```python
from build123d import *

# Parameters (mm, degrees)
F0_R      = 25.4
F1_DEPTH  = 95.25
F2_R      = 25.4
F2_R_2    = 19.05
F3_DEPTH  = 38.1
F4_R      = 25.4
F4_R_2    = 19.05
F5_DEPTH  = 38.1
F7_DEPTH  = 12.7
F9_DEPTH  = 46.228
F10_R     = 4.826
F11_DEPTH = 22.352


with BuildPart() as f1:
    # F0 (on Right) → F1 (new body)
    with BuildSketch(Plane.YZ):
        Circle(F0_R)
    extrude(amount=F1_DEPTH)

    # F2 (on face) → F3 (cut)
    with BuildSketch(Plane.YZ.offset(95.25)):
        Circle(F2_R)
        Circle(F2_R_2, mode=Mode.SUBTRACT)
    extrude(amount=-F3_DEPTH, mode=Mode.SUBTRACT)

    # F4 (on face) → F5 (cut)
    with BuildSketch(Plane(origin=(0, 0, 0), x_dir=(0, -1, 0), z_dir=(-1, 0, 0))):
        Circle(F4_R)
        Circle(F4_R_2, mode=Mode.SUBTRACT)
    extrude(amount=-F5_DEPTH, mode=Mode.SUBTRACT)

    # F6 (on face) → F7 (cut)
    with BuildSketch(Plane(origin=(0, 0, 0), x_dir=(0, -1, 0), z_dir=(-1, 0, 0))):
        with BuildLine():
            ThreePointArc((6.35, 17.9605122421), (3.2213926947, 18.7756525614), (0, 19.05))
            ThreePointArc((0, 19.05), (-3.2213926947, 18.7756525614), (-6.35, 17.9605122421))
            Line((-6.35, 17.9605122421), (-6.35, -17.9605122421))
            ThreePointArc((-6.35, -17.9605122421), (-3.2213926947, -18.7756525614), (0, -19.05))
            ThreePointArc((0, -19.05), (3.2213926947, -18.7756525614), (6.35, -17.9605122421))
            Line((6.35, -17.9605122421), (6.35, 17.9605122421))
        make_face()
    extrude(amount=-F7_DEPTH, mode=Mode.SUBTRACT)

    # F8 (on face) → F9 (cut)
    with BuildSketch(Plane.YZ.offset(95.25)):
        with BuildLine():
            Line((-40.058898566, 25.4), (-40.058898566, 21.5428465581))
            Line((-40.058898566, 21.5428465581), (-40.058898566, 12.7))
            Line((-40.058898566, 12.7), (-14.1990316571, 12.7))
            ThreePointArc((-14.1990316571, 12.7), (0, 19.05), (14.1990316571, 12.7))
            Line((14.1990316571, 12.7), (36.141101434, 12.7))
            Line((36.141101434, 12.7), (36.141101434, 25.4))
            Line((36.141101434, 25.4), (-40.058898566, 25.4))
        make_face()
        with BuildLine():
            ThreePointArc((14.1990316571, 12.7), (0, 19.05), (-14.1990316571, 12.7))
            Line((-14.1990316571, 12.7), (14.1990316571, 12.7))
        make_face()
    extrude(amount=-F9_DEPTH, mode=Mode.SUBTRACT)

    # F10 (on face) → F11 (cut)
    with BuildSketch(Plane.XY.offset(12.7)):
        with Locations((76.2, 0)):
            Circle(F10_R)
    extrude(amount=-F11_DEPTH, mode=Mode.SUBTRACT)


solid = f1.part
```
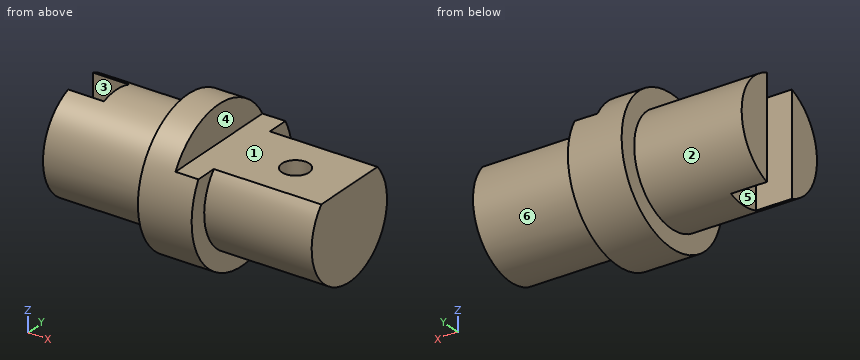
Read the model definition and answer for the solid it produces. Units are mm, in the model's axes. Face numbers are marked on the shaded views. A direction names the side the tool comes from. Give positions to 0.01 mm unless a question says otherwise; leave off trailing zeros. Loops run counter-clockwise (first coordinate to the right, second up) from the corner with the lowest first, then second, coordinate; pieces in that order, holes last.
Item 1: The part is cut by section A-A (z = 0). Write down the section's boundary in (x, y).
Item 2: For the marked faces 4, 5 and 6, determine the directions among +Z, -Z, +X, -X, +Y, -Y from which every point of the face is accessible in a straight line to the end or side of a thin tool.
Item 3: Each of these flat-tipped pins is pushed along its axis until it touches: pin 1 Ø8.5 at (x, y) = (76.2, 0) entering from +Z; pin 2 Ø14 at (x, z) = (3.5, 0) entering from -Y; pin 3 Ø10.5 at (x, y) = (77, -1) entering from +Z. Where does it stop, or does it pass through?
Item 4: Find the intervals of material crossed by line 1 along X through (y, z) = (21.5, -3); line 2 along Y through (x, z) = (15, -0.5); line 3 along Y through (x, z) = (76, -4), in increasing order.
Item 5: The part is cut by section C-C (y = 0). Write down the section's boundary in (x, z).
Item 6: The mould has two halves that part along Y. Classify the marked faces 1, 2 and 3: released by +Y, released by -Y, zero draft, split by the parting line, or undercut.
Item 7: The part is cut by section D-D (z = -11.5). Write down the section's boundary in (x, y), and give its area (3 significant figures).
Item 8: The part is cut by section B-B (x = 7.5). Write down the section's boundary in (y, z), and give its area (3 significant figures).
Taken from the geometry:
1. outline: (0, -19.05) - (38.1, -19.05) - (38.1, -25.4) - (57.15, -25.4) - (57.15, -19.05) - (95.25, -19.05) - (95.25, 19.05) - (57.15, 19.05) - (57.15, 25.4) - (38.1, 25.4) - (38.1, 19.05) - (0, 19.05) - (0, 6.35) - (12.7, 6.35) - (12.7, -6.35) - (0, -6.35) - close; hole circle Ø9.65 at (76.2, 0)
2. face 4: +Z, +X, +Y, -Y
2. face 5: +Z, -Z, -X
2. face 6: +X
3. pin 1: stops at z = -9.65
3. pin 2: stops at y = -19.05
3. pin 3: stops at z = 12.7
4. line 1: x = 38.1 to 57.15
4. line 2: y = -19.04 to 19.04
4. line 3: y = -18.63 to -4.82, 4.82 to 18.63
5. outline: (12.7, -19.05) - (38.1, -19.05) - (38.1, -25.4) - (57.15, -25.4) - (57.15, -19.05) - (95.25, -19.05) - (95.25, 12.7) - (81.03, 12.7) - (81.03, -9.65) - (71.37, -9.65) - (71.37, 12.7) - (49.02, 12.7) - (49.02, 25.4) - (38.1, 25.4) - (38.1, 19.05) - (12.7, 19.05) - close
6. face 1: zero draft
6. face 2: split by the parting line
6. face 3: undercut
7. outline: (0, -15.19) - (38.1, -15.19) - (38.1, -22.65) - (57.15, -22.65) - (57.15, -15.19) - (95.25, -15.19) - (95.25, 15.19) - (57.15, 15.19) - (57.15, 22.65) - (38.1, 22.65) - (38.1, 15.19) - (0, 15.19) - (0, 6.35) - (12.7, 6.35) - (12.7, -6.35) - (0, -6.35) - close
7. area: 3,020 mm2
8. outline: (-6.35, -17.96) - (-6.35, 17.96) arc R19.05 ccw to start; (6.35, -17.96) arc R19.05 ccw to (6.35, 17.96) - close
8. area: 665 mm2
